Check sheet for the modelled part. Datum: model origin and axes. Units: mm. A direction names the side the tool comes from. Give positions to 0.01 mm unless a question says otherwise; leave off trailing zeros. Order: outer loops, then holes, each group sorted by start corner. A loop starts at its lowest first (then second) coordinate and runs counter-clockwise, first axis right, second up.
```python
from build123d import *

# Parameters (mm, degrees)
SKETCH033_W     = 101.85
SKETCH033_H     = 58.42
PAD011_DEPTH    = 1.2
SKETCH034_W     = 6.366
SKETCH034_H     = 6.811
POCKET017_DEPTH = 1.201
SKETCH035_R     = 1.25
POCKET018_DEPTH = 1.201
SKETCH036_R     = 6
PAD012_DEPTH    = 5
SKETCH037_W     = 6.84
SKETCH037_H     = 6.4
SKETCH037_W_2   = 6.94
PAD013_DEPTH    = 7.2
SKETCH039_W     = 17.01
SKETCH039_H     = 21.96
PAD014_DEPTH    = 5
SKETCH038_W     = 15.16
SKETCH038_H     = 16.61
PAD015_DEPTH    = 2
SKETCH040_W     = 4.49
SKETCH040_H     = 7.51
PAD016_DEPTH    = 4


with BuildPart() as part:
    # Sketch033 → Pad011 (new body)
    with BuildSketch(Plane.XY):
        with Locations((50.925, 29.21)):
            Rectangle(SKETCH033_W, SKETCH033_H)
    extrude(amount=PAD011_DEPTH)

    # Sketch034 (on Face6 of Pad011) → Pocket017 (cut, through all)
    with BuildSketch(Plane.XY.offset(1.2)):
        with Locations((3.183, 55.0145)):
            Rectangle(SKETCH034_W, SKETCH034_H)
        with Locations((98.667, 55.0145)):
            Rectangle(SKETCH034_W, SKETCH034_H)
        with Locations((98.667, 3.4055)):
            Rectangle(SKETCH034_W, SKETCH034_H)
        with Locations((3.183, 3.4055)):
            Rectangle(SKETCH034_W, SKETCH034_H)
    extrude(amount=-POCKET017_DEPTH, mode=Mode.SUBTRACT)

    # Sketch035 (on Face4 of Pocket017) → Pocket018 (cut, through all)
    with BuildSketch(Plane.XY.offset(1.2)):
        with Locations((5.105, 47.625)):
            Circle(SKETCH035_R)
        with Locations((94.564, 47.625)):
            Circle(SKETCH035_R)
        with Locations((94.564, 10.795)):
            Circle(SKETCH035_R)
        with Locations((5.105, 10.795)):
            Circle(SKETCH035_R)
    extrude(amount=-POCKET018_DEPTH, mode=Mode.SUBTRACT)

    # Sketch036 (on Face4 of Pocket018) → Pad012 (join)
    with BuildSketch(Plane.XY.offset(1.2)):
        with Locations((90, 20.2)):
            Circle(SKETCH036_R)
    extrude(amount=PAD012_DEPTH)

    # Sketch037 (on Face4 of Pocket018) → Pad013 (join)
    with BuildSketch(Plane.XY.offset(1.2)):
        with Locations((28.8, 4.33)):
            Rectangle(SKETCH037_W, SKETCH037_H)
        with Locations((77.7, 4.33)):
            Rectangle(SKETCH037_W_2, SKETCH037_H)
    extrude(amount=PAD013_DEPTH)

    # Sketch039 (on Face4 of Pocket018) → Pad014 (join)
    with BuildSketch(Plane.XY.offset(1.2)):
        with Locations((19.775, 46.78)):
            Rectangle(SKETCH039_W, SKETCH039_H)
    extrude(amount=PAD014_DEPTH)

    # Sketch038 (on Face4 of Pocket018) → Pad015 (join)
    with BuildSketch(Plane.XY.offset(1.2)):
        with Locations((38.83, 49.785)):
            Rectangle(SKETCH038_W, SKETCH038_H)
    extrude(amount=PAD015_DEPTH)

    # Sketch040 (on Face4 of Pad015) → Pad016 (join)
    with BuildSketch(Plane.XY.offset(1.2)):
        with Locations((1.645, 28.025)):
            Rectangle(SKETCH040_W, SKETCH040_H)
    extrude(amount=PAD016_DEPTH)


with BuildPart() as part_1:
    # Body004 placement: moved
    add(part.part.moved(Location((0, 0, 4))))


solid = part_1.part
```
Q1. Tool access check on faces 1 (the cylindrical face through (85.58, 24.26, 7.66)), 2 (the flat face through (3.89, 28, 7)), 3 (the flat face through (78, 1.13, 9)), 4 (the flat face through (20, 57.76, 8)). Record the directions out of +Z, -Z, +X, -X, +Y, -Y that give a thin tool (end or side, any length) a straight path to the whole face; none if there is none.
Q2. Draft check along X on faces 5 (the flat face through (2, 28, 9.2)), 6 (the flat face through (28.28, 47, 8)), 7 (the flat face through (46.41, 50, 6)). Enter one of: pulls with the +X half, pulls with the -X half, needs draft (parallel to the pull), parting line crosses it, or undercut.
Q3. Sectioned sample at B-B, the plane y = 20.2. Record the cut outline in (x, z), plus the area to 3 significant figures.
Q4. Sectioned sample at D-D, the plane y = 33. Record the cut outline in (x, z).
Q5. Sectioned sample at A-A, the plane z = 8.25. Record the cut outline in (x, y).
Q6. Material ranges on line 1 (X direction, y = 46, z = 5.75); line 2 (Z direction, x = 82, y = 30); line 3 (Z direction, x = 85.5, y = 22), recorded low to high.
Q7. Go/stop test with flat-tipped pins: P1, Ø1.3, axis at x = 100, z = 4.5, coming from the -Y side; P2, Ø1.6, axis at y = 51, z = 6.5, coming from the +X side; P3, Ø3.5, axis at x = 77.5, z = 7, coming from the -Y side. Record where each tip stops, or that it passes through.
Q8. Sectioned sample at C-C, the plane x = 77.5. Record the cut outline in (y, z), plus the area to 3 significant figures.
Filled in:
1. face 1: +Z
1. face 2: +Z, +Y, -Y
1. face 3: +Z, +X, -X, -Y
1. face 4: +Z, -X, +Y
2. face 5: needs draft
2. face 6: undercut
2. face 7: pulls with the +X half
3. outline: (0, 4) - (101.85, 4) - (101.85, 5.2) - (96, 5.2) - (96, 10.2) - (84, 10.2) - (84, 5.2) - (0, 5.2) - close
3. area: 182 mm2
4. outline: (0, 4) - (101.85, 4) - (101.85, 5.2) - (0, 5.2) - close
5. outline: (-0.6, 24.27) - (3.89, 24.27) - (3.89, 31.78) - (-0.6, 31.78) - close; (11.27, 35.8) - (28.28, 35.8) - (28.28, 57.76) - (11.27, 57.76) - close; (25.38, 1.13) - (32.22, 1.13) - (32.22, 7.53) - (25.38, 7.53) - close; (74.23, 1.13) - (81.17, 1.13) - (81.17, 7.53) - (74.23, 7.53) - close; circle Ø12 at (90, 20.2)
6. line 1: x = 11.27 to 28.28, 31.25 to 46.41
6. line 2: z = 4 to 5.2
6. line 3: z = 4 to 10.2
7. P1: stops at y = 6.81
7. P2: stops at x = 46.41
7. P3: stops at y = 1.13
8. outline: (0, 4) - (58.42, 4) - (58.42, 5.2) - (7.53, 5.2) - (7.53, 12.4) - (1.13, 12.4) - (1.13, 5.2) - (0, 5.2) - close
8. area: 116 mm2
